Here's how the part is built. I have some questions about the finished solid (model axes, mm). Face numbers are marked on the shaded views. A direction names the side the tool comes from. Round coordinates to 2 decimals unless told otherwise and drop trailing zeros. Write each loop counter-clockwise with the first axis right and the second up, starting at its lowest first coordinate (ties: lowest second). Pieces come first, ordered by that corner, then holes. Notation, with made-up numbers: (78.5, 80) -> (123.5, 80) arc R18 cw to (123.5, 97) -> close; hole circle Ø4 at (89.25, -24). An arc over 180 degrees is marked (long way). Put each result on its own line as item: value. Start each with the question number.
1. Suppose I cut it at A-A (x = 0). Please give me the cut outline in (y, z).
2. Suppose I cut it at D-D (z = 2.75). Please give me the cut outline in (x, y).
3. Which directions (+Z, -Z, +X, -X, +Y, -Y) give clear straight access to the entire face, cutting with the end or side of a thin tool? Please do the marked faces 5 and 6.
4. I need wall thicknesses on probe 1 along X at (y, z) = (0, 6.75); probe 2 along X at (y, z) = (1, 6.5). Which ranges of each line are inside material? Lowest first, please. Write a range as from..to.
5. Suppose I cut it at B-B (z = 8.25). Please give me the cut outline in (x, y).
6. We'd pull the mould along Y, two halves only. Please class the marked faces 1, 2, 3 and 4: +Y half, -Y half, draft (parallel to the pull), parting line (faces both ways), or undercut.
7. Suppose I cut it at C-C (y = 15). Please give me the cut outline in (x, z), then the cut area to 3 significant figures.
8. For pin 1 (3.5 mm diameter, centred on x = -0.5, y = 15, fed in from +Z); pin 2 (1.5 mm diameter, centred on x = 15, z = 9, fed in from +Y); pin 3 (2 mm diameter, centred on y = -7.5, z = 7.5, fed in from -X), each with a flat end and sliding along its axis, tell me the tip position at first contact or that it passes through.
Solid Edge part; units mm, degrees
sketch "Sketch1" plane through (0, 0, 0) normal (0, 0, 1) x (1, 0, 0)
  circle A0 centre (0, 0) radius 13
  circle A1 centre (0, 0) radius 17
extrude "Protrusion1" add sketch "Sketch1" along normal blind 10
hole "Hole_1" at (0, -15, 0) direction (0, 0, 1) diameter 2.7 end up to next
sketch "Sketch2" plane through (0, 0, 10) normal (0, 0, 1) x (-1, 0, 0)
  line L0 (-2.75, 12.7058) -> (2.75, 12.7058)
  line L1 (2.75, 12.7058) -> (2.75, 17.7796)
  line L2 (2.75, 17.7796) -> (-2.75, 17.7796)
  line L3 (-2.75, 17.7796) -> (-2.75, 16.7761)
extrude "ExtrudedCutout_1" cut sketch "Sketch2" against normal blind 3 material side at (0, -12.7558, 10)
pattern_circular "Pattern2" count 4 over 360 about axis through (0, 0, 0) along (0, 0, 1) of "Hole_1", "ExtrudedCutout_1"
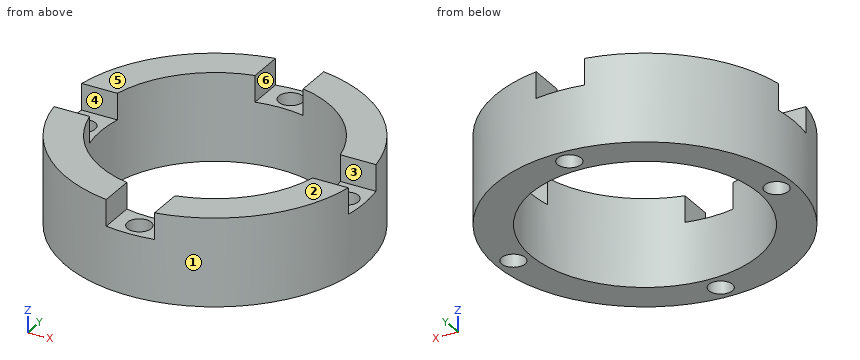
Verdict:
1. outline: (-17, 0) -> (-16.35, 0) -> (-16.35, 7) -> (-17, 7) -> close; (-13.65, 0) -> (-13, 0) -> (-13, 7) -> (-13.65, 7) -> close; (13, 0) -> (13.65, 0) -> (13.65, 7) -> (13, 7) -> close; (16.35, 0) -> (17, 0) -> (17, 7) -> (16.35, 7) -> close
2. outline: circle Ø34 at (0, 0); hole circle Ø2.7 at (-15, 0); hole circle Ø26 at (0, 0); hole circle Ø2.7 at (0, -15); hole circle Ø2.7 at (0, 15); hole circle Ø2.7 at (15, 0)
3. face 5: +Z, +X, -X, +Y, -Y
3. face 6: +Z, +Y, -Y
4. probe 1: x = -17..-16.35, -13.65..-13, 13..13.65, 16.35..17
4. probe 2: x = -16.97..-15.91, -14.09..-12.96, 12.96..14.09, 15.91..16.97
5. outline: (-16.78, -2.75) arc R17 ccw to (-2.75, -16.78) -> (-2.75, -12.71) arc R13 cw to (-12.71, -2.75) -> close; (-16.78, 2.75) -> (-12.71, 2.75) arc R13 cw to (-2.75, 12.71) -> (-2.75, 16.78) arc R17 ccw to start; (2.75, -16.78) arc R17 ccw to (16.78, -2.75) -> (12.71, -2.75) arc R13 cw to (2.75, -12.71) -> close; (2.75, 12.71) arc R13 cw to (12.71, 2.75) -> (16.78, 2.75) arc R17 ccw to (2.75, 16.78) -> close
6. face 1: parting line
6. face 2: draft
6. face 3: undercut
6. face 4: undercut
7. outline: (-8, 0) -> (-1.35, 0) -> (-1.35, 7) -> (-2.75, 7) -> (-2.75, 10) -> (-8, 10) -> close; (1.35, 0) -> (8, 0) -> (8, 10) -> (2.75, 10) -> (2.75, 7) -> (1.35, 7) -> close
7. area: 125 mm^2
8. pin 1: stops at z = 7
8. pin 2: stops at y = 9.27
8. pin 3: stops at x = -15.71
